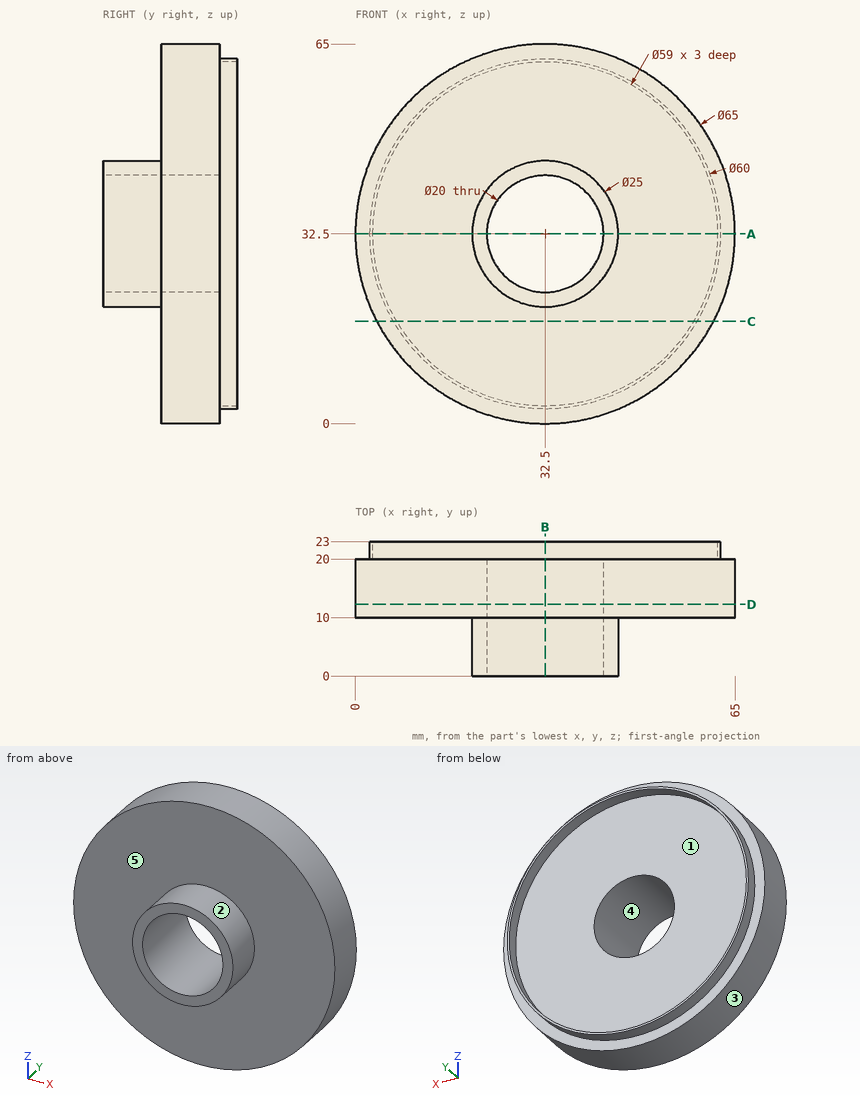
The figure shows three views and two pictorial views of one solid part (mm, origin at its lowest corner). Answer the questions. A direction names the side the tool comes from. Round coordinates to 2 decimals unless told otherwise and drop trailing zeros. Loops run counter-clockwise (first coordinate to the right, second up) from the corner with the lowest first, then second, coordinate; pieces in that order, holes last. Notation, with made-up numbers: M -21,1 L 29,1 A32 cw 29,29 Z; hole C 8.25,-2 d5. An arc over 180 degrees is marked long. Return JSON: item names as keys, results as strings.
Q1. Find section A-A, the plane z = 32.5. Determine the outline of the cut face in (x, y), plus the area to 3 significant figures.
Results list:
{"outline": "M 0,10 L 20,10 L 20,0 L 22.5,0 L 22.5,20 L 3,20 L 3,23 L 2.5,23 L 2.5,20 L 0,20 Z; M 42.5,0 L 45,0 L 45,10 L 65,10 L 65,20 L 62.5,20 L 62.5,23 L 62,23 L 62,20 L 42.5,20 Z", "area": "503 mm2"}
Q2. Each of these flat-tipped pins is pushed along its axis until it touches: pin 1 Ø2 at (y, z) = (20, 41) entering from -X; pin 2 Ø4 at (x, y) = (35.5, 15.5) entering from +Z; pin 3 Ø5 at (x, y) = (17.5, 11) entering from +Z; pin 4 Ø18 at (x, z) = (32.5, 32.5) entering from +Y. Where does it stop, or does it pass through?
Results list:
{"pin 1": "stops at x = 0.88", "pin 2": "stops at z = 64.98", "pin 3": "stops at z = 62.5", "pin 4": "passes through"}
Q3. Find section B-B, the plane x = 32.5. Determine the outline of the cut face in (y, z), plus the area to 3 significant figures.
Results list:
{"outline": "M 0,20 L 10,20 L 10,0 L 20,0 L 20,2.5 L 23,2.5 L 23,3 L 20,3 L 20,22.5 L 0,22.5 Z; M 0,42.5 L 20,42.5 L 20,62 L 23,62 L 23,62.5 L 20,62.5 L 20,65 L 10,65 L 10,45 L 0,45 Z", "area": "503 mm2"}
Q4. The mould has two halves that part along X. Classify the marked faces 3, 4 and 5: released by +X, released by -X, zero draft, split by the parting line, or undercut.
Results list:
{"face 3": "split by the parting line", "face 4": "undercut", "face 5": "zero draft"}
Q5. Which of the six approach directions +Z, -Z, +X, -X, +Y, -Y give full straight-line access (tool end or side, diameter ignored) to the marked faces 1 and 2?
Results list:
{"face 1": "+Y", "face 2": "-Y"}
Q6. Find the intervals of material crossed by line 1 along Z through (x, y) = (32.5, 7.25); line 2 along Y through (x, z) = (43, 10); line 3 along Z through (x, y) = (32.5, 22.4), in increasing order. Write a range as from..to.
Results list:
{"line 1": "z = 20..22.5, 42.5..45", "line 2": "y = 10..20", "line 3": "z = 2.5..3, 62..62.5"}
Q7. Find section C-C, the plane z = 17.5. Determine the outline of the cut face in (x, y), plus the area to 3 significant figures.
Results list:
{"outline": "M 3.67,10 L 61.33,10 L 61.33,20 L 58.48,20 L 58.48,23 L 57.9,23 L 57.9,20 L 7.1,20 L 7.1,23 L 6.52,23 L 6.52,20 L 3.67,20 Z", "area": "580 mm2"}
Q8. Find section D-D, the plane y = 12.25. Determine the outline of the cut face in (x, z).
Results list:
{"outline": "C 32.5,32.5 d65; hole C 32.5,32.5 d20"}
